from build123d import *
from build123d.topology import SkipClean

# Parameters (mm, degrees)
BOSS_EXTRUDE1_DEPTH     = 30
CUT_EXTRUDE1_DEPTH      = 5
CUT_EXTRUDE1_DEPTH_BACK = 5
SKETCH2_R               = 4
CUT_EXTRUDE2_START      = -3
CUT_EXTRUDE2_DEPTH      = 3


with BuildPart() as part:
    # Sketch1 → Boss-Extrude1 (new body)
    with BuildSketch(Plane(origin=(0, 0, 0), x_dir=(-1, 0, 0), z_dir=(0, 0, 1))):
        with BuildLine():
            Line((0, 0), (10, 0))
            ThreePointArc((10, 0), (23.5, 13.5), (37, 0))
            Line((37, 0), (153.995672066, 0))
            Line((153.995672066, 0), (176.985, 0))
            ThreePointArc((176.985, 0), (180.985, 4), (184.985, 0))
            Line((184.985, 0), (194.985, 0))
            ThreePointArc((194.985, 0), (190.884494937, 9.899494937), (180.985, 14))
            Line((180.985, 14), (23.5, 23.5))
            ThreePointArc((23.5, 23.5), (6.882990642, 16.617009358), (0, 0))
        make_face()
    boss_extrude1 = extrude(amount=BOSS_EXTRUDE1_DEPTH)

    # Mirror1: Boss-Extrude1 across Top Plane
    with SkipClean():  # the faces are left unmerged after this step: merging them gives an invalid solid
        add(boss_extrude1.mirror(Plane(origin=(0, 0, 0), x_dir=(1, 0, 0), z_dir=(0, 1, 0))))

    # Sketch2 → Cut-Extrude1 (cut, two sides: drawn at the far end of the back side and taken through both)
    with SkipClean():  # the faces are left unmerged after this step: merging them gives an invalid solid
        with BuildSketch(Plane.XY.offset(15).offset(-CUT_EXTRUDE1_DEPTH_BACK)):
            with BuildLine():
                Line((-145.016260464, 16.169749662), (-180.985, 14))
                ThreePointArc((-180.985, 14), (-194.985, 0), (-180.985, -14))
                Line((-180.985, -14), (-145.016260464, -16.169749662))
                Line((-145.016260464, -16.169749662), (-145.016260464, 16.169749662))
            make_face()
            with Locations(Location((-180.985, 0, 0), (0, 0, 180))):
                Circle(SKETCH2_R, mode=Mode.SUBTRACT)
        extrude(amount=CUT_EXTRUDE1_DEPTH + CUT_EXTRUDE1_DEPTH_BACK, mode=Mode.SUBTRACT)

    # Sketch3 → Cut-Extrude2 (cut)
    with SkipClean():  # the faces are left unmerged after this step: merging them gives an invalid solid
        with BuildSketch(Plane.XY.offset(30).offset(CUT_EXTRUDE2_START)):
            with BuildLine():
                Line((-171.779614491, 10.548027191), (-37.825745268, 18.628553956))
                ThreePointArc((-37.825745268, 18.628553956), (-47, 0), (-37.825745268, -18.628553956))
                Line((-37.825745268, -18.628553956), (-171.779614491, -10.548027191))
                ThreePointArc((-171.779614491, -10.548027191), (-166.985, 0), (-171.779614491, 10.548027191))
            make_face()
        cut_extrude2 = extrude(amount=CUT_EXTRUDE2_DEPTH, mode=Mode.SUBTRACT)

    # Mirror2: Cut-Extrude2 across plane
    with SkipClean():  # the faces are left unmerged after this step: merging them gives an invalid solid
        add(cut_extrude2.mirror(Plane.XY.offset(15)), mode=Mode.SUBTRACT)


solid = part.part
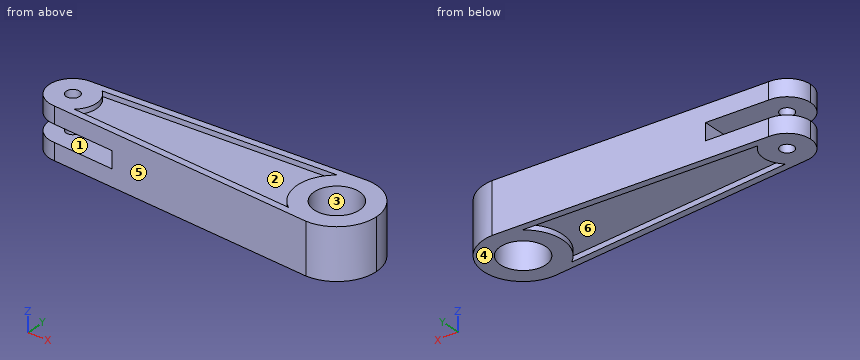
Part model, mm, in its own coordinate system. Face numbers are marked on the shaded views. A direction names the side the tool comes from. Coordinates: 2 decimals unless noted, no trailing zeros. Loops run counter-clockwise (first coordinate to the right, second up) from the corner with the lowest first, then second, coordinate; pieces in that order, holes last. Notation, with made-up numbers: M 25,79.5 L 40,79.5 A17 cw 40,100.5 Z; hole C 82,-26.75 d4. An arc over 180 degrees is marked long. Use a Markdown table: item, result. Add a question column.
Q1. Pin check, flat tips, straight feed: P1, Ø12, axis at y = -4.5, z = 8.5, coming from the +X side; P2, Ø1.5, axis at x = -29, z = 4, coming from the +Y side; P3, Ø2, axis at x = -107.5, z = 23.5, coming from the +Y side; P4, Ø8, axis at x = -30.5, y = -3.5, coming from the -Z side. Stop position of each tip, or through.
Q2. Which spindle directions (+Z, -Z, +X, -X, +Y, -Y) get a long thin tool onto all of the face, cutting with end or side? Do the marked faces 1, 2 and 3. Say none if no direction does.
Q3. Cut at B-B (y = 7.5). Write the cut outline in (x, z).
Q4. Cut at D-D (x = -162.5). Write the cut outline in (y, z).
Q5. Mould opens along Y. For the marked faces 4, 5 and 6 say: +Y half, -Y half, draft (parallel to the pull), parting line (faces both ways), or undercut.
Q6. Cut at C-C (z = 16). Write the cut outline in (x, y), and give its area (3 significant figures).
Q7. Probe L1, parallel to X at y = 0, z = 23.25 (3 decimals); L2, parallel to X at y = 0, z = 27.25 (3 decimals); L3, parallel to X at y = 0, z = 11. List the from-to ranges inside material, lowest first.
Q8. Cut at A-A (z = 7.75). Write the cut outline in (x, y) (3 decimals).
Worked out:
| question | item | result |
|---|---|---|
| 1 | P1 | stops at x = 0 |
| 1 | P2 | stops at y = 23.21 |
| 1 | P3 | stops at y = 18.49 |
| 1 | P4 | passes through |
| 2 | face 1 | -X, +Y, -Y |
| 2 | face 2 | +Z |
| 2 | face 3 | +Z, -Z |
| 3 | outline | M -192.81,0 L -169.16,0 L -169.16,3 L -45.77,3 L -45.77,0 L -34.72,0 L -34.72,30 L -45.77,30 L -45.77,27 L -169.16,27 L -169.16,30 L -192.81,30 L -192.81,20 L -145.02,20 L -145.02,10 L -192.81,10 Z; M -12.28,0 L -1.23,0 L -1.23,30 L -12.28,30 Z |
| 4 | outline | M -15.12,0 L -11.11,0 L -11.11,3 L 11.11,3 L 11.11,0 L 15.12,0 L 15.12,10 L -15.12,10 Z; M -15.12,20 L 15.12,20 L 15.12,30 L 11.11,30 L 11.11,27 L -11.11,27 L -11.11,30 L -15.12,30 Z |
| 5 | face 4 | draft |
| 5 | face 5 | -Y half |
| 5 | face 6 | undercut |
| 6 | outline | M -145.02,-16.17 L -23.5,-23.5 A23.5 ccw -23.5,23.5 L -145.02,16.17 Z; hole C -23.5,0 d27 |
| 6 | area | 5,120 mm2 |
| 7 | L1 | x = -194.985 to -184.985, -176.985 to -37, -10 to 0 |
| 7 | L2 | x = -194.985 to -184.985, -176.985 to -166.985, -47 to -37, -10 to 0 |
| 7 | L3 | x = -145.02 to -37, -10 to 0 |
| 8 | outline | M -180.985,-14 L -23.5,-23.5 A23.5 ccw -23.5,23.5 L -180.985,14 A14 ccw Z; hole C -180.985,0 d8; hole C -23.5,0 d27 |
